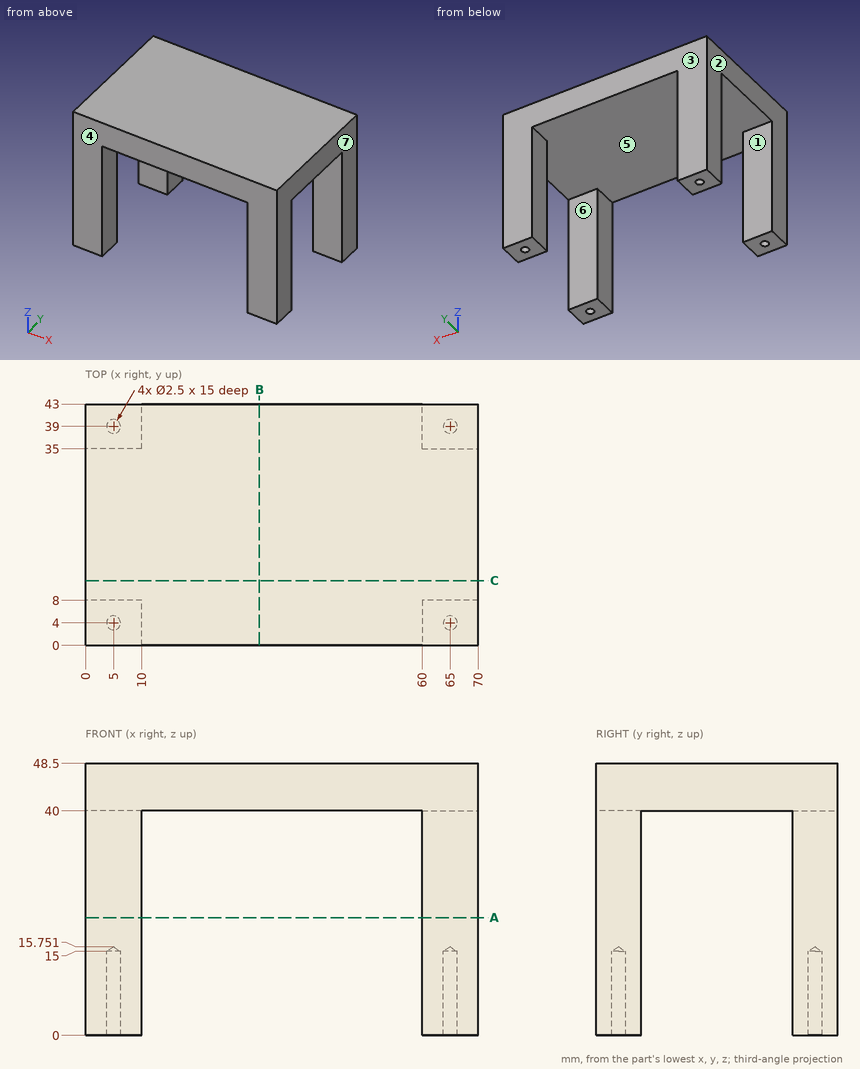
Here's the drawing with two shaded views (mm, measured from the low corner). I have some questions. A direction names the side the tool comes from. Give positions to 0.01 mm unless a question says otherwise; leave off trailing zeros. Order: outer loops, then holes, each group sorted by start corner. A loop starts at its lowest first (then second) coordinate and runs counter-clockwise, first axis right, second up. Notation, with made-up numbers: M 49.25,6.5 L 95.25,6.5 A24 cw 95.25,45.5 Z; hole C 25.5,76.25 d9. An arc over 180 degrees is marked long. Answer as a JSON object with one key per item and string values. Group by question number.
1) We'd pull the mould along Y, two halves only. Please class the marked faces 1, 2, 3 and 4: pulls with the +Y half, pulls with the -Y half, needs draft (parallel to the pull), parting line crosses it, or undercut.
2) Suppose I cut it at A-A, the plane z = 21. Write out the boundary of the cut face in (x, y), plus the area to 3 significant figures.
3) On a 3-axis mill with a long thin cutter (end or side, diameter ignored), from which of +Z, -Z, +X, -X, +Y, -Y can I reach the whole of each face in a straight line? I mean the marked faces 5, 6 and 7. Say none if no direction works.
4) Suppose I cut it at C-C, the plane y = 11.5. Write out the boundary of the cut face in (x, z), plus the area to 3 significant figures.
5) I'm going to push flat-ended pins straight in: pin 1 Ø10 at (x, z) = (30.5, 31) entering from +Y; pin 2 Ø13 at (x, y) = (40.5, 23) entering from -Z; pin 3 Ø1.5 at (x, y) = (65, 4) entering from -Z. Where does each tip first touch, or does it pass through?
6) Suppose I cut it at B-B, the plane x = 31. Write out the boundary of the cut face in (y, z), plus the area to 4 significant figures.
7) Please list where these lines run through material, in increasing order: L1, parallel to X at y = 4, z = 7; L2, parallel to Y at x = 65, z = 6.5; L3, parallel to X at y = 7, z = 20. Write a range as [from, to].
Results found:
{
 "1": {"face 1": "undercut", "face 2": "needs draft", "face 3": "pulls with the +Y half", "face 4": "pulls with the -Y half"},
 "2": {"outline": "M 0,0 L 10,0 L 10,8 L 0,8 Z; M 0,35 L 10,35 L 10,43 L 0,43 Z; M 60,0 L 70,0 L 70,8 L 60,8 Z; M 60,35 L 70,35 L 70,43 L 60,43 Z", "area": "320 mm²"},
 "3": {"face 5": "-Z", "face 6": "-Z, +X, -X", "face 7": "+Z, -Z, +X, +Y, -Y"},
 "4": {"outline": "M 0,40 L 70,40 L 70,48.5 L 0,48.5 Z", "area": "595 mm²"},
 "5": {"pin 1": "through", "pin 2": "z = 40", "pin 3": "z = 15.3"},
 "6": {"outline": "M 0,40 L 43,40 L 43,48.5 L 0,48.5 Z", "area": "365.5 mm²"},
 "7": {"L1": "[0, 3.75], [6.25, 10], [60, 63.75], [66.25, 70]", "L2": "[0, 2.75], [5.25, 8], [35, 37.75], [40.25, 43]", "L3": "[0, 10], [60, 70]"}
}
